Autodesk Inventor part; units mm, degrees
ref_plane "YZ Plane" through (0, 0, 0) normal (1, 0, 0) x (0, 1, 0)
ref_plane "XZ Plane" through (0, 0, 0) normal (0, 1, 0) x (-1, 0, 0)
ref_plane "XY Plane" through (0, 0, 0) normal (0, 0, 1) x (1, 0, 0)
sketch "Sketch1" plane through (0, 0, 0) normal (0, 1, 0) x (-1, 0, 0)
  line L0 (0, 0) -> (0, -7)
  line L1 (0, -7) -> (2.5, -7)
  line L2 (2.5, -7) -> (2.5, -2.5)
  line L3 (2.5, -2.5) -> (7, -2.5)
  line L4 (7, -2.5) -> (7, 0)
  line L5 (7, 0) -> (0, 0)
  line L6 (0, -30) -> (0, -23)
  line L7 (0, -23) -> (2.5, -23)
  line L8 (2.5, -23) -> (2.5, -27.5)
  line L9 (2.5, -27.5) -> (7, -27.5)
  line L10 (7, -27.5) -> (7, -30)
  line L11 (7, -30) -> (0, -30)
  line L12 (23, 0) -> (30, 0)
  line L13 (30, 0) -> (30, -7)
  line L14 (30, -7) -> (27.5, -7)
  line L15 (27.5, -7) -> (27.5, -2.5)
  line L16 (27.5, -2.5) -> (23, -2.5)
  line L17 (23, -2.5) -> (23, 0)
  line L18 (30, -23) -> (30, -30)
  line L19 (30, -30) -> (23, -30)
  line L20 (23, -30) -> (23, -27.5)
  line L21 (23, -27.5) -> (27.5, -27.5)
  line L22 (27.5, -27.5) -> (27.5, -23)
  line L23 (27.5, -23) -> (30, -23)
  dimension "d0" = 7
  dimension "d1" = 2.5
  dimension "d2" = 4.5
  dimension "d3" = 4.5
  dimension "d8" = 7
  dimension "d9" = 4.5
  dimension "d10" = 7
  dimension "d11" = 7
  dimension "d12" = 2.5
  dimension "d13" = 30
  dimension "d14" = 30
  dimension "d15" = 30
  dimension "d16" = 2.5
  dimension "d17" = 2.5
  dimension "d18" = 4.5
  dimension "d19" = 7
extrude "Extrusion1" add sketch "Sketch1" along normal blind 25
sketch "Sketch2" plane through (0, 0, 0) normal (0, -1, 0) x (1, 0, 0)
  line L0 (0, 0) -> (-30, 0)
  line L1 (-30, 0) -> (-30, -30)
  line L2 (-30, -30) -> (0, -30)
  line L3 (0, -30) -> (0, 0)
  line L4 (-27.5, -2.5) -> (-2.5, -2.5)
  line L5 (-2.5, -2.5) -> (-2.5, -27.5)
  line L6 (-2.5, -27.5) -> (-27.5, -27.5)
  line L7 (-27.5, -27.5) -> (-23, -27.5)
  line L8 (-27.5, -27.5) -> (-27.5, -2.5)
extrude "Extrusion2" add sketch "Sketch2" against normal blind 7
sketch "Sketch3" plane through (0, 25, 0) normal (0, 1, 0) x (1, 0, 0)
  line L0 (0, 0) -> (-7, 0)
  line L1 (0, 0) -> (-30, 0)
  line L2 (-7, 0) -> (-7, 7)
  line L3 (-7, 7) -> (0, 7)
  line L4 (0, 7) -> (0, 0)
  line L5 (0, 30) -> (-7, 30)
  line L6 (-7, 30) -> (-7, 23)
  line L7 (-7, 23) -> (0, 23)
  line L8 (-2.5, 23) -> (0, 23)
  line L9 (0, 23) -> (0, 30)
  line L10 (0, 23) -> (0, 30)
  line L11 (-30, 30) -> (-30, 23)
  line L12 (-30, 0) -> (-30, 30)
  line L13 (-30, 23) -> (-23, 23)
  line L14 (-23, 23) -> (-23, 30)
  line L15 (-23, 30) -> (-30, 30)
  line L16 (-30, 30) -> (0, 30)
  line L17 (-30, 0) -> (-23, 0)
  line L18 (-23, 0) -> (-23, 7)
  line L19 (-23, 7) -> (-30, 7)
  line L20 (-27.5, 7) -> (-30, 7)
  line L21 (-30, 7) -> (-30, 0)
  dimension "d24" = 7
  dimension "d25" = 7
  dimension "d26" = 7
  dimension "d27" = 7
  dimension "d28" = 7
extrude "Extrusion3" add sketch "Sketch3" along normal blind 1
sketch "Sketch4" plane through (0, 0, 0) normal (1, 0, 0) x (0, 0, -1)
  line L0 (0, 0) -> (7, 0)
  line L1 (27.5, 0) -> (2.5, 0)
  line L2 (7, 0) -> (7, 2)
  line L3 (7, 2) -> (0, 2)
  line L4 (0, 2) -> (0, 0)
  line L5 (30, 0) -> (30, 2)
  line L6 (30, 0) -> (30, 26)
  line L7 (30, 2) -> (23, 2)
  line L8 (23, 2) -> (23, 0)
  line L9 (0, 0) -> (30, 0)
  line L10 (23, 0) -> (30, 0)
  dimension "d31" = 7
  dimension "d32" = 2
  dimension "d33" = 2
  dimension "d34" = 7
sketch "Sketch5" plane through (0, 0, -30) normal (0, 0, -1) x (-1, 0, 0)
  line L0 (0, 0) -> (7, 0)
  line L1 (7, 0) -> (7, 2)
  line L2 (7, 2) -> (0, 2)
  line L3 (0, 2) -> (0, 0)
  line L4 (30, 0) -> (30, 2)
  line L5 (30, 0) -> (30, 26)
  line L6 (30, 2) -> (23, 2)
  line L7 (23, 2) -> (23, 0)
  line L8 (23, 0) -> (30, 0)
  line L9 (30, 0) -> (0, 0)
  dimension "d35" = 7
  dimension "d36" = 2
  dimension "d37" = 2
  dimension "d38" = 7
extrude "Extrusion4" add sketch "Sketch4" along normal blind 7
extrude "Extrusion5" add sketch "Sketch5" along normal blind 7
sketch "Sketch6" plane through (0, 2, 0) normal (0, 1, 0) x (1, 0, 0)
  circle A0 centre (3.5, 3.5) radius 2
  line L0 (7, 7) -> (7, 0)
  line L1 (0, 0) -> (7, 0)
  point P0 (7, 3.5)
  point P1 (3.5, 0)
  dimension "d43" = 4
sketch "Sketch7" plane through (0, 2, -23) normal (0, 1, 0) x (1, 0, 0)
  circle A0 centre (3.5, 3.5) radius 2
  line L0 (7, 7) -> (7, 0)
  line L1 (0, 0) -> (7, 0)
  point P0 (0, -23)
  point P1 (7, 3.5)
  point P2 (3.5, 0)
  dimension "d44" = 4
sketch "Sketch8" plane through (-7, 2, -30) normal (0, 1, 0) x (1, 0, 0)
  circle A0 centre (3.5, 3.5) radius 2
  circle A1 centre (-19.5, 3.5) radius 2
  line L0 (7, 0) -> (7, 7)
  line L1 (7, 0) -> (0, 0)
  line L2 (-23, 0) -> (-23, 7)
  line L3 (-23, 7) -> (-16, 7)
  point P0 (7, -30)
  point P1 (7, 3.5)
  point P2 (3.5, 0)
  point P3 (-23, 3.5)
  point P4 (-19.5, 7)
  dimension "d45" = 4
  dimension "d46" = 4
extrude "Extrusion6" cut sketch "Sketch6" against normal blind 2
extrude "Extrusion7" cut sketch "Sketch7" against normal blind 2
extrude "Extrusion8" cut sketch "Sketch8" against normal blind 2
sketch "Sketch9" plane through (0, 25, 0) normal (0, -1, 0) x (1, 0, 0)
  line L0 (0, -30) -> (0, 0)
  line L1 (0, 0) -> (-30, 0)
  line L2 (-30, 0) -> (-30, -30)
  line L3 (-30, 0) -> (-30, -37)
  line L4 (-2.5, -2.5) -> (-2.5, -27.5)
  line L5 (-2.5, -27.5) -> (-27.5, -27.5)
  line L6 (-27.5, -27.5) -> (-23, -27.5)
  line L7 (-27.5, -27.5) -> (-27.5, -2.5)
  line L8 (-27.5, -2.5) -> (-2.5, -2.5)
  line L9 (-2.5, -2.5) -> (-7, -2.5)
  line L10 (0, -30) -> (-30, -30)
extrude "Extrusion9" add sketch "Sketch9" along normal blind 6 and the other way blind 1
sketch "Sketch10" plane through (-30, 0, 0) normal (-1, 0, 0) x (0, 0, 1)
  line L0 (0, 0) -> (-11.5, 0)
  line L1 (0, 0) -> (-37, 0)
  line L2 (-11.5, 0) -> (-18.5, 0)
  line L3 (-27.5, 0) -> (-2.5, 0)
  line L4 (-18.5, 0) -> (-30, 0)
  line L5 (-18.5, 0) -> (-18.5, 7)
  line L6 (-7, 7) -> (-23, 7)
  line L7 (-11.5, 0) -> (-11.5, 7)
  line L8 (-18.5, 7) -> (-11.5, 7)
  line L9 (-11.5, 0) -> (-11.5, -7)
  line L10 (-11.5, -7) -> (-18.5, -7)
  line L11 (-18.5, -7) -> (-18.5, 0)
  dimension "d57" = 11.5
  dimension "d58" = 7
  dimension "d59" = 7
extrude "Extrusion10" add sketch "Sketch10" along normal blind 2
sketch "Sketch11" plane through (-30, 26, 0) normal (0, 0, 1) x (1, 0, 0)
  line L0 (0, -26) -> (11.5, -26)
  line L1 (2.5, -26) -> (27.5, -26)
  line L2 (11.5, -26) -> (18.5, -26)
  line L3 (18.5, -26) -> (18.5, -33)
  line L4 (18.5, -33) -> (11.5, -33)
  line L5 (11.5, -33) -> (11.5, -26)
  line L6 (23, -19) -> (7, -19)
  line L7 (11.5, -19) -> (18.5, -19)
  line L8 (18.5, -26) -> (18.5, -19)
  line L9 (11.5, -26) -> (11.5, -19)
  point P0 (30, -26)
  dimension "d62" = 11.5
  dimension "d63" = 7
  dimension "d64" = 7
extrude "Extrusion11" add sketch "Sketch11" along normal blind 2
sketch "Sketch12" plane through (-32, 0, 0) normal (-1, 0, 0) x (0, 0, 1)
  circle A0 centre (-15, -3.5) radius 2
  line L0 (-18.5, -7) -> (-11.5, -7)
  line L1 (-11.5, -7) -> (-11.5, 0)
  point P0 (0, 0)
  point P1 (-15, -7)
  point P2 (-11.5, -3.5)
  dimension "d67" = 4
sketch "Sketch13" plane through (-30, 26, 2) normal (0, 0, 1) x (1, 0, 0)
  circle A0 centre (15, -29.5) radius 2
  line L0 (11.5, -26) -> (11.5, -33)
  line L1 (11.5, -33) -> (18.5, -33)
  point P0 (30, -26)
  point P1 (11.5, -29.5)
  point P2 (15, -33)
  dimension "d68" = 4
extrude "Extrusion12" cut sketch "Sketch12" against normal blind 2
extrude "Extrusion13" cut sketch "Sketch13" against normal blind 2
properties part number "ygolki" material "Bronze, Soft Tin"
Geometry: final body of the model. Coordinates: model frame, mm. A direction names the side the tool comes from. Coordinates: 2 decimals unless noted, no trailing zeros. Order: outer loops, then holes, each group sorted by start corner. A loop starts at its lowest first (then second) coordinate and runs counter-clockwise, first axis right, second up.
1) Set-up query: faces 1 (the flat face through (-11.5, 0, 1)), 2 (the flat face through (-1, 13, -23)), 3 (the flat face through (-25.3, 25.5, -7)). Return all of +Z, -Z, +X, -X, +Y, -Y with unobstructed straight access to the full face (end or side cutting, diameter ignored); none if empty.
Result sheet:
face 1: +Z, +X, +Y, -Y
face 2: +X, -X
face 3: +Y, -Y
2) Ray query, probe 1 along Z at (x, y) = (3.5, 0.45); probe 2 along Z at (x, y) = (-29, 13.5); probe 3 along Y at (x, z) = (-15, 0.9). Return the intervals inside material, ascending.
Result sheet:
probe 1: z = -30 to -28.5, -24.5 to -23, -7 to -5.5, -1.5 to 0
probe 2: z = -30 to -23, -7 to 0
probe 3: y = -7 to -5.5, -1.5 to 7
3) First-contact query: P1, Ø10, axis at x = -2, z = -9.5, coming from the -Y side; P2, Ø10, axis at y = 4.5, z = -5.5, coming from the -X side; P3, Ø0.8, axis at x = -1.5, y = 15.5, coming from the -Z side; P4, Ø3.5, axis at x = 3.5, z = -26.5, coming from the -Y side. Flat tips, straight axial feed; report the tip coordinate or a pass-through.
Result sheet:
P1: stops at y = 0
P2: stops at x = -30
P3: stops at z = -30
P4: passes through
4) Section D-D (z = -26.5). Return loops of the section in (x, y), then the cut area to 3 significant figures.
Result sheet:
outline: (-30, 0) - (-27.5, 0) - (-27.5, 25) - (-23, 25) - (-23, 26) - (-30, 26) - close; (-7, 25) - (-2.5, 25) - (-2.5, 0) - (1.5, 0) - (1.5, 2) - (0, 2) - (0, 26) - (-7, 26) - close; (5.5, 0) - (7, 0) - (7, 2) - (5.5, 2) - close
area: 145 mm2
5) Section A-A (x = 3.5). Return loops of the section in (y, z), then the cut area to 3 significant figures.
Result sheet:
outline: (0, -30) - (2, -30) - (2, -28.5) - (0, -28.5) - close; (0, -24.5) - (2, -24.5) - (2, -23) - (0, -23) - close; (0, -7) - (2, -7) - (2, -5.5) - (0, -5.5) - close; (0, -1.5) - (2, -1.5) - (2, 0) - (0, 0) - close
area: 12.0 mm2
6) Draft query along X for faces 4 (the flat face through (-7, 13, -1)), 5 (the flat face through (-30, -5, -17)), 6 (the flat face through (-3, 1, -37)). Return one class per face: released by +X, released by -X, zero draft, split by the parting line, or undercut.
Result sheet:
face 4: undercut
face 5: released by +X
face 6: zero draft
7) Section C-C (y = 6). Return loops of the section in (x, z).
Result sheet:
outline: (-32, -18.5) - (-30, -18.5) - (-30, -30) - (0, -30) - (0, 0) - (-11.5, 0) - (-11.5, 2) - (-18.5, 2) - (-18.5, 0) - (-30, 0) - (-30, -11.5) - (-32, -11.5) - close; hole (-27.5, -27.5) - (-2.5, -27.5) - (-2.5, -2.5) - (-27.5, -2.5) - close
8) Section B-B (z = -10.5). Return loops of the section in (x, y), then the cut area to 3 significant figures.
Result sheet:
outline: (-30, 0) - (-27.5, 0) - (-27.5, 7) - (-30, 7) - close; (-30, 19) - (-27.5, 19) - (-27.5, 26) - (-30, 26) - close; (-2.5, 0) - (0, 0) - (0, 7) - (-2.5, 7) - close; (-2.5, 19) - (0, 19) - (0, 26) - (-2.5, 26) - close
area: 70.0 mm2
